The figure shows three views and two pictorial views of one solid part (mm, origin at its lowest corner). Answer the questions. A direction names the side the tool comes from. Coordinates: 2 decimals unless noted, no trailing zeros. Write each loop counter-clockwise with the first axis right and the second up, starting at its lowest first coordinate (ties: lowest second). Pieces come first, ordered by that corner, then holes.
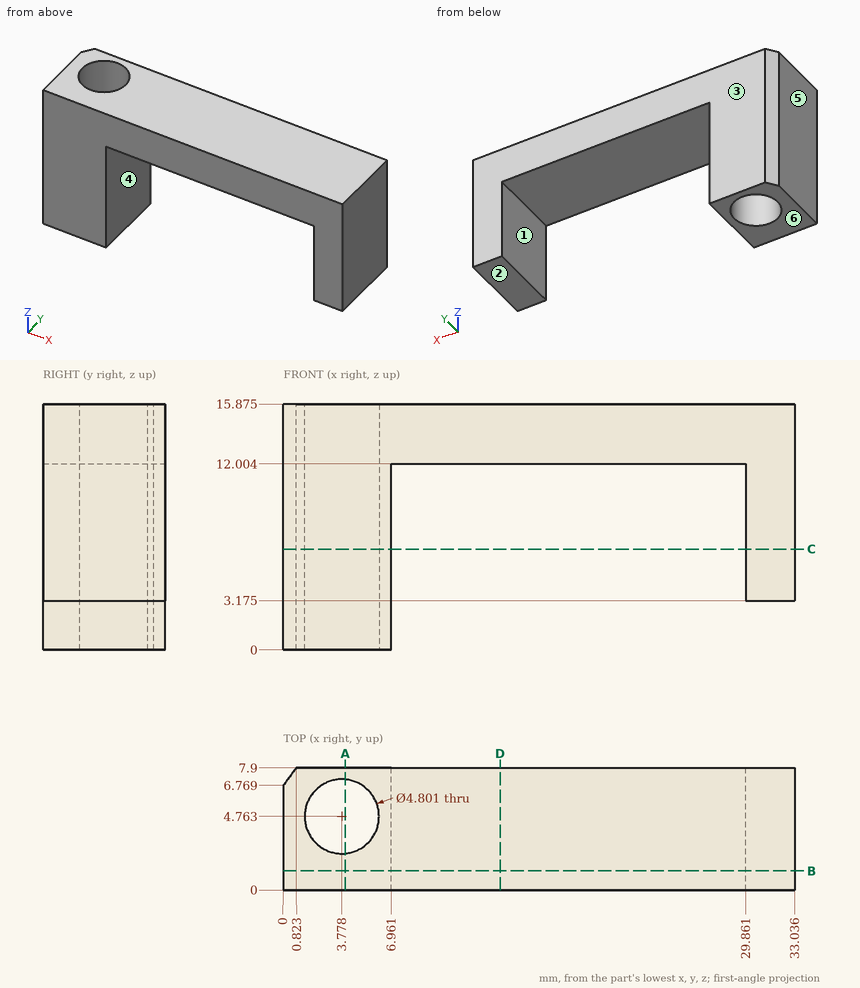
Item 1: Given pin 1 (3 mm diameter, centred on x = 4.5, z = 5, fed in from -Y); pin 2 (1 mm diameter, centred on x = 31.5, y = 5, fed in from -Z) (1 decimal), each flat-ended and moving along its own axis, determine where each tip first touches the part or whether it passes through.
Item 2: The part is cut by section B-B (y = 1.25). Give the vertices of the cut face in (x, z) (1 decimal).
Item 3: The part is cut by section A-A (x = 4). Give the vertices of the cut face in (y, z) (1 decimal).
Item 4: The part is cut by section D-D (x = 14). Give the vertices of the cut face in (y, z) (1 decimal), and give its area (3 significant figures).
Item 5: Determine the mould class of the marked faces 4, 5 and 6 for opening direction X: +X half, -X half, draft (parallel to the pull), parting line (faces both ways), or undercut.
Item 6: For the marked faces 1, 2 and 3, determine the directions among +Z, -Z, +X, -X, +Y, -Y from which every point of the face is accessible in a straight line to the end or side of a thin tool.
Item 7: The part is cut by section C-C (z = 6.5). Give the vertices of the cut face in (x, y).
Item 8: Find the intervals of material crossed by probe 1 along X at (y, z) = (4.75, 15); probe 2 along X at (y, z) = (2.75, 11.5) (1 decimal); probe 3 along X at (y, z) = (3.25, 4.75) (1 decimal), in increasing order.
Answer:
1. pin 1: stops at y = 0
1. pin 2: stops at z = 3.2
2. outline: (0, 0) - (7, 0) - (7, 12) - (29.9, 12) - (29.9, 3.2) - (33, 3.2) - (33, 15.9) - (0, 15.9) - close
3. outline: (0, 0) - (2.4, 0) - (2.4, 15.9) - (0, 15.9) - close; (7.2, 0) - (7.9, 0) - (7.9, 15.9) - (7.2, 15.9) - close
4. outline: (0, 12) - (7.9, 12) - (7.9, 15.9) - (0, 15.9) - close
4. area: 30.6 mm2
5. face 4: undercut
5. face 5: -X half
5. face 6: draft
6. face 1: -Z, +Y, -Y
6. face 2: -Z, +X, +Y, -Y
6. face 3: +Z, -Z, +X, -X, +Y
7. outline: (0, 0) - (6.96, 0) - (6.96, 7.9) - (0.82, 7.9) - (0, 6.77) - close; (29.86, 0) - (33.04, 0) - (33.04, 7.9) - (29.86, 7.9) - close; hole circle Ø4.8 at (3.78, 4.76)
8. probe 1: x = 0 to 1.38, 6.18 to 33.04
8. probe 2: x = 0 to 2.5, 5.1 to 7, 29.9 to 33
8. probe 3: x = 0 to 1.9, 5.6 to 7, 29.9 to 33
